Can you work these out from the model? Positions are in its coordinate system, mm. A direction names the side the tool comes from. Give positions to 0.01 mm unless a question says otherwise; leave off trailing zeros. Loops run counter-clockwise (first coordinate to the right, second up) from the corner with the lowest first, then second, coordinate; pieces in that order, holes last. Notation, with made-up numbers: M 72.25,2.5 L 128.25,2.5 A27 cw 128.25,28.5 Z; hole C -11,26 d2. An arc over 180 degrees is marked long. Put each result on its own line as item: value. Start each with the question number.
1) Imagine slicing it at A-A (x = 10.25). Write out the boundary of the cut face in (y, z), then the cut area to 3 significant figures.
2) Imagine slicing it at B-B (z = 8). Write out the boundary of the cut face in (x, y), then the cut area to 3 significant figures.
3) For P1, Ø6, axis at y = 6, z = 4, coming from the +X side; P2, Ø3.5, axis at x = 18, z = 8.5, coming from the -Y side; P3, Ø5, axis at x = 20, z = 6.5, coming from the -Y side, each with a flat end and sliding along its axis, tell me the tip position at first contact or that it passes through.
4) Imagine slicing it at C-C (y = 4.75). Write out the boundary of the cut face in (x, z), then the cut area to 4 significant figures.
5) If we mould it in two halves opening along Y, with no side actions, what happens to faces 5 (the flat face through (24.5, 18.5, 6.2)), 6 (the flat face through (12, 19, 6)), 7 (the cylindrical face through (14.199, 8.035, 6.162))? For each: +Y half, -Y half, draft (parallel to the pull), parting line (faces both ways), or undercut.
6) Imagine slicing it at D-D (x = 16.75). Write out the boundary of the cut face in (y, z), then the cut area to 4 significant figures.
7) Please list where these lines run through material, in increasing order: line 1 along Y through (x, z) = (10.25, 3); line 2 along X through (y, z) = (5.5, 9); line 3 along Y through (x, z) = (23, 10.25). Write a range as from..to.
8) For faces 1 (the cylindrical face through (21.86, 17.138, 6.162)), 2 (the flat face through (23, 17, 6)), 3 (the cylindrical face through (14.215, 2.699, 6.162)), 4 (the flat face through (7, 2.5, 6)), which set-ups out of +Z, -Z, +X, -X, +Y, -Y let a thin tool reach every point of the face, with its end or its side?
from build123d import *

# Parameters (mm, degrees)
SKETCH1_W           = 3
SKETCH1_H           = 0.5
BOSS_EXTRUDE1_DEPTH = 12.5
FILLET1_R           = 1


with BuildPart() as part:
    # Sketch1 → Boss-Extrude1 (new body)
    with BuildSketch(Plane.XY):
        Polygon((14.5, 17.5), (14.5, 7.75), (2.5, 7.75), (2.5, 2.5), (14.5, 2.5), (14.5, 0), (0, 0), (0, 19), (24.5, 19), (24.5, 17.5), align=None)
        with Locations((23, 17.25)):
            Rectangle(SKETCH1_W, SKETCH1_H)
        with Locations((13, 2.75)):
            Rectangle(SKETCH1_W, SKETCH1_H)
    extrude(amount=BOSS_EXTRUDE1_DEPTH)

    # Fillet1
    # the kernel refuses this fillet: 1 mm, written as the material it takes off along each edge
    with BuildSketch(Plane(origin=(24.5, 17, -2.5), x_dir=(-1, 0, 0), z_dir=(0, 0, 1)), Plane(origin=(14.5, 3, -2.5), x_dir=(0, -1, 0), z_dir=(0, 0, 1))) as fillet1_piece_1:
        with BuildLine():
            CenterArc((FILLET1_R, -FILLET1_R), FILLET1_R, 90, 90)
            Line((0, -FILLET1_R), (-FILLET1_R * 0.02, -FILLET1_R))
            Line((-FILLET1_R * 0.02, -FILLET1_R), (-FILLET1_R * 0.02, FILLET1_R * 0.02))
            Line((-FILLET1_R * 0.02, FILLET1_R * 0.02), (FILLET1_R, FILLET1_R * 0.02))
            Line((FILLET1_R, FILLET1_R * 0.02), (FILLET1_R, 0))
        make_face()
    extrude(amount=17.5, mode=Mode.SUBTRACT)
    with BuildSketch(Plane(origin=(21.5, 17, -2.165063509), x_dir=(0, 1, 0), z_dir=(0, 0, 1))) as fillet1_piece_2:
        with BuildLine():
            CenterArc((1, -0.866025404), FILLET1_R, 120, 60)
            Line((0, -0.866025404), (-0.02, -0.866025404))
            Line((-0.02, -0.866025404), (-0.02, 0))
            Line((-0.02, 0), (0, 0.02))
            ThreePointArc((0, 0.02), (0.25, 0.02), (0.49, 0.017320508))
            Line((0.49, 0.017320508), (0.5, 0))
        make_face()
    extrude(amount=16.830127019, mode=Mode.SUBTRACT)
    with BuildSketch(Plane(origin=(11.5, 3, -2.165063509), x_dir=(1, 0, 0), z_dir=(0, 0, 1))) as fillet1_piece_3:
        with BuildLine():
            CenterArc((0.866025404, -1), FILLET1_R, 90, 60)
            Line((0, -0.5), (-0.017320508, -0.49))
            ThreePointArc((-0.017320508, -0.49), (-0.02, -0.25), (-0.02, 0))
            Line((-0.02, 0), (0, 0.02))
            Line((0, 0.02), (0.866025404, 0.02))
            Line((0.866025404, 0.02), (0.866025404, 0))
        make_face()
    extrude(amount=16.830127019, mode=Mode.SUBTRACT)
    with BuildSketch(Plane(origin=(14.5, 7.75, -2.5), x_dir=(0, 1, 0), z_dir=(0, 0, 1))) as fillet1_piece_4:
        with BuildLine():
            CenterArc((FILLET1_R, FILLET1_R), FILLET1_R, 180, 90)
            Line((0, FILLET1_R), (-FILLET1_R * 0.02, FILLET1_R))
            Line((-FILLET1_R * 0.02, FILLET1_R), (-FILLET1_R * 0.02, -FILLET1_R * 0.02))
            Line((-FILLET1_R * 0.02, -FILLET1_R * 0.02), (FILLET1_R, -FILLET1_R * 0.02))
            Line((FILLET1_R, -FILLET1_R * 0.02), (FILLET1_R, 0))
        make_face()
    extrude(amount=17.5, mode=Mode.SUBTRACT)


solid = part.part
Recorded:
1. outline: M 0,0 L 2.5,0 L 2.5,12.5 L 0,12.5 Z; M 7.75,0 L 19,0 L 19,12.5 L 7.75,12.5 Z
1. area: 172 mm²
2. outline: M 0,0 L 14.5,0 L 14.5,2 A1 ccw 13.5,3 L 12.37,3 A1 ccw 11.5,2.5 L 2.5,2.5 L 2.5,7.75 L 13.5,7.75 A1 ccw 14.5,8.75 L 14.5,17.5 L 21.5,17.5 A1 ccw 22.37,17 L 23.5,17 A1 ccw 24.5,18 L 24.5,19 L 0,19 Z
2. area: 230 mm²
3. P1: x = 14.5
3. P2: y = 17.5
3. P3: y = 17
4. outline: M 0,0 L 2.5,0 L 2.5,12.5 L 0,12.5 Z
4. area: 31.25 mm²
5. face 5: draft
5. face 6: +Y half
5. face 7: undercut
6. outline: M 17.5,0 L 19,0 L 19,12.5 L 17.5,12.5 Z
6. area: 18.75 mm²
7. line 1: 0..2.5, 7.75..19
7. line 2: 0..2.5
7. line 3: 17..19
8. face 1: +Z, -Z, -Y
8. face 2: +Z, -Z, +X, -Y
8. face 3: +Z, -Z, +X
8. face 4: +Z, -Z
